```python
from build123d import *

# Parameters (mm, degrees)
EXTRUDE1_DEPTH = 3
SKETCH2_R      = 1.5875
EXTRUDE2_DEPTH = 3
SKETCH4_R      = 1.59
EXTRUDE3_DEPTH = 3
SKETCH5_R      = 1.59
EXTRUDE5_DEPTH = 3


with BuildPart() as part:
    # Sketch1 → Extrude1 (new body)
    with BuildSketch(Plane(origin=(0, 0, 0), x_dir=(1, 0, 0), z_dir=(0, 1, 0))):
        Polygon((0, 0), (-145, 0), (-145, -20), (-24, -20), (0, -20), align=None)
    extrude(amount=EXTRUDE1_DEPTH)

    # Sketch2 → Extrude2 (cut)
    with BuildSketch(Plane(origin=(0, 3, 0), x_dir=(1, 0, 0), z_dir=(0, 1, 0))):
        with Locations(Location((-139, -7.5, 0), (0, 0, 270))):
            Circle(SKETCH2_R)
        with Locations(Location((-7.2248, -7.5, 0), (0, 0, 270))):
            Circle(SKETCH2_R)
        with Locations((-7.2248, -99.358338)):
            Circle(SKETCH2_R)
    extrude(amount=-EXTRUDE2_DEPTH, mode=Mode.SUBTRACT)

    # Sketch4 → Extrude3 (cut)
    with BuildSketch(Plane(origin=(0, 3, 0), x_dir=(1, 0, 0), z_dir=(0, 1, 0))):
        with Locations(Location((-21.5348, -7.5, 0), (0, 0, 270))):
            Circle(SKETCH4_R)
    extrude(amount=-EXTRUDE3_DEPTH, mode=Mode.SUBTRACT)

    # Sketch5 → Extrude5 (cut)
    with BuildSketch(Plane(origin=(0, 3, 0), x_dir=(1, 0, 0), z_dir=(0, 1, 0))):
        with Locations(Location((-129.5348, -17.71, 0), (0, 0, 270))):
            Circle(SKETCH5_R)
    extrude(amount=-EXTRUDE5_DEPTH, mode=Mode.SUBTRACT)


solid = part.part
```
Work out the finished part from the listing and answer in its coordinate system (mm). Give positions to 0.01 mm unless a question says otherwise; leave off trailing zeros. Loops run counter-clockwise (first coordinate to the right, second up) from the corner with the lowest first, then second, coordinate; pieces in that order, holes last. Notation, with made-up numbers: (79, 12.25) - (98, 12.25) arc R18 ccw to (98, 21.25) - close; hole circle Ø11 at (17.25, 32.5). An arc over 180 degrees is marked (long way). Use CSV: the item, a comma, the result in double quotes. Start each with the question number.
(1) Each of these flat-tipped pins is pushed along its axis until it touches: pin 1 (5 mm diameter, centred on x = -21.53, z = 7.5, fed in from +Y); pin 2 (3 mm diameter, centred on x = -139, z = 7.5, fed in from +Y). Where does it stop, or does it pass through?
(2) Find section B-B, the plane z = 17.71. Determine the outline of the cut face in (x, y).
(3) Find the intervals of material crossed by L1, parallel to X at y = 0.85, z = 7.5; L2, parallel to Z at x = -139, y = 0.7; L3, parallel to X at y = 0.75, z = 17.71, in increasing order.
(4) Find section C-C, the plane z = 7.5. Determine the outline of the cut face in (x, y), plus the area to 3 significant figures.
(5) Determine the mould class of faces 1 (the face through (-74, 1, 20)), 2 (the face through (-74, 3, 10)), 3 (the face through (-140.55, 1.52, 7.16)) for opening direction Z: released by +Z, released by -Z, zero draft, split by the parting line, or undercut.
(6) Find section A-A, the plane x = -139. Determine the outline of the cut face in (y, z), plus the area to 3 significant figures.
Results found:
1,pin 1,"y = 3"
1,pin 2,"through"
2,outline,"(-145, 0) - (-131.12, 0) - (-131.12, 3) - (-145, 3) - close; (-127.94, 0) - (0, 0) - (0, 3) - (-127.94, 3) - close"
3,L1,"-145 to -140.59, -137.41 to -23.12, -19.94 to -8.81, -5.64 to 0"
3,L2,"0 to 5.91, 9.09 to 20"
3,L3,"-145 to -131.12, -127.94 to 0"
4,outline,"(-145, 0) - (-140.59, 0) - (-140.59, 3) - (-145, 3) - close; (-137.41, 0) - (-23.12, 0) - (-23.12, 3) - (-137.41, 3) - close; (-19.94, 0) - (-8.81, 0) - (-8.81, 3) - (-19.94, 3) - close; (-5.64, 0) - (0, 0) - (0, 3) - (-5.64, 3) - close"
4,area,"406 mm^2"
5,face 1,"released by +Z"
5,face 2,"zero draft"
5,face 3,"undercut"
6,outline,"(0, 0) - (3, 0) - (3, 5.91) - (0, 5.91) - close; (0, 9.09) - (3, 9.09) - (3, 20) - (0, 20) - close"
6,area,"50.5 mm^2"
